from build123d import *

# Parameters (mm, degrees)
SKETCH1_W              = 190.5
SKETCH1_H              = 209.55
BOSS_EXTRUDE2_DEPTH    = 5.08
SKETCH2_R              = 8.73125
CUT_EXTRUDE1_DEPTH     = 6.08
F_10_CLEARANCE_HOLE2_D = 5.1054
FILLET1_R              = 4.445
F_10_CLEARANCE_HOLE1_D = 5.1054


with BuildPart() as part:
    # Sketch1 → Boss-Extrude2 (new body)
    with BuildSketch(Plane(origin=(0, 0, 0), x_dir=(0, 0, -1), z_dir=(1, 0, 0))):
        with Locations((95.25, 104.775)):
            Rectangle(SKETCH1_W, SKETCH1_H)
    extrude(amount=BOSS_EXTRUDE2_DEPTH)

    # Sketch2 → Cut-Extrude1 (cut, through all)
    with BuildSketch(Plane(origin=(5.08, 0, 0), x_dir=(0, 0, -1), z_dir=(1, 0, 0))):
        with Locations((95.25, 50.8)):
            Circle(SKETCH2_R)
    extrude(amount=-CUT_EXTRUDE1_DEPTH, mode=Mode.SUBTRACT)

    # #10 Clearance Hole2 (through all)
    with Locations(Plane(origin=(5.08, 0, 0), x_dir=(0, 0, -1), z_dir=(1, 0, 0))):
        with Locations((53.975, 28.575), (53.975, 155.575), (161.925, 155.575), (161.925, 28.575)):
            Hole(F_10_CLEARANCE_HOLE2_D / 2)

    # Fillet1
    fillet1_edges = [part.edges().sort_by_distance(p)[0] for p in [
        (2.54, 209.55, 0),
        (2.54, 209.55, -190.5),
        (2.54, 0, -190.5),
        (2.54, 0, 0),
    ]]
    fillet(fillet1_edges, radius=FILLET1_R)

    # #10 Clearance Hole1 (through all)
    with Locations(Plane(origin=(5.08, 0, 0), x_dir=(0, 0, -1), z_dir=(1, 0, 0))):
        with Locations((6.35, 203.2), (184.15, 6.35), (6.35, 6.35), (184.15, 203.2), (95.25, 6.35), (95.25, 203.2), (6.35, 137.583333333), (6.35, 71.966666667), (184.15, 71.966666667), (184.15, 137.583333333)):
            Hole(F_10_CLEARANCE_HOLE1_D / 2)


solid = part.part
Model file for the job. Use its own axes, mm. Give positions to 0.01 mm unless a question says otherwise; leave off trailing zeros. Loops run counter-clockwise (first coordinate to the right, second up) from the corner with the lowest first, then second, coordinate; pieces in that order, holes last.
Item 1: Drop a flat-ended pin along its axis: P1, Ø6, axis at y = 6.35, z = -184.15, coming from the -X side. Give the stop position or say it passes through.
Check values:
P1: stops at x = 0
Item 2: Slice it at A-A (y = 50.8). Write the cut outline in (x, z).
Check values:
outline: (0, -190.5) - (5.08, -190.5) - (5.08, -103.98) - (0, -103.98) - close; (0, -86.52) - (5.08, -86.52) - (5.08, 0) - (0, 0) - close
Item 3: Mould opens along Y. For faces 1 (the face through (2.576, 208.282, -189.163)), 2 (the face through (2.504, 30.3, -55.856)), 3 (the face through (2.5, 135.09, -6.9)), 4 (the face through (2.576, 1.337, -1.268)) say: +Y half, -Y half, draft (parallel to the pull), parting line (faces both ways), or undercut.
Check values:
face 1: +Y half
face 2: undercut
face 3: undercut
face 4: -Y half
Item 4: Drill centre lines: line 1 along Y through (x, z) = (3.25, -184.15); line 2 along Z through (x, y) = (3, 203.2); line 3 along Y through (x, z) = (2.5, -7.5). Where is each one in solid material? Low to high.
Check values:
line 1: y = 0 to 3.8, 8.9 to 69.41, 74.52 to 135.03, 140.14 to 200.65, 205.75 to 209.55
line 2: z = -190.5 to -186.7, -181.6 to -97.8, -92.7 to -8.9, -3.8 to 0
line 3: y = 0 to 4.07, 8.63 to 69.69, 74.25 to 135.3, 139.86 to 200.92, 205.48 to 209.55
Item 5: Slice it at B-B (z = -95.25). Write the cut outline in (x, y), plus the area to 3 significant figures.
Check values:
outline: (0, 0) - (5.08, 0) - (5.08, 3.8) - (0, 3.8) - close; (0, 8.9) - (5.08, 8.9) - (5.08, 42.07) - (0, 42.07) - close; (0, 59.53) - (5.08, 59.53) - (5.08, 200.65) - (0, 200.65) - close; (0, 205.75) - (5.08, 205.75) - (5.08, 209.55) - (0, 209.55) - close
area: 924 mm2
